Here's how the part is built. I have some questions about the finished solid (model axes, mm). A direction names the side the tool comes from. Round coordinates to 2 decimals unless told otherwise and drop trailing zeros. Write each loop counter-clockwise with the first axis right and the second up, starting at its lowest first coordinate (ties: lowest second). Pieces come first, ordered by that corner, then holes. Notation, with made-up numbers: M 27.5,53.25 L 31.5,53.25 A34 ccw 31.5,83.25 Z; hole C 40,-15.75 d6. An arc over 180 degrees is marked long. Write item = value, one per line. Start each with the question number.
(1) I want a section at C-C (y = -13). List the corners of the cut face in (x, z) for me.
(2) I want a section at D-D (z = 4). List the corners of the cut face in (x, y) for me, and give its area (3 significant figures).
(3) I need wall thicknesses on line 1 along X through (y, z) = (-9.5, 8.5); line 2 along X through (y, z) = (-25.5, 5.5); line 3 along Y through (x, z) = (-3, 8.25). Which ranges of each line are inside material? Lowest first, please.
(4) I want a section at B-B (x = 6.5). List the corners of the cut face in (y, z) for me, and give its area (3 significant figures).
(5) I want a section at A-A (z = 8.5). List the corners of the cut face in (x, y) for me, and give its area (3 significant figures).
(6) Will these pins go through, and if not, where does the flat tip stop? pin 1 Ø5 at (x, y) = (36.5, -15.5) entering from +Z; pin 2 Ø1.5 at (x, z) = (26, 5.5) entering from -Y; pin 3 Ø4 at (x, z) = (-6, 1.5) entering from +Y.
(7) If we mould it in two halves opening along X, with no side actions, what happens to faces 4 (the flat face through (-10.06, -39.96, 4.93)), 5 (the flat face through (27.17, -20.175, 7.465)), 6 (the flat face through (19, -15, 0))? For each: released by +X, released by -X, zero draft, split by the parting line, or undercut.
(8) On a 3-axis mill with a long thin cutter (end or side, diameter ignored), from which of +Z, -Z, +X, -X, +Y, -Y can I reach the whole of each face in a straight line? I mean faces 1 (the cylindrical face through (38.06, 5.15, 7.46)), 2 (the flat face through (-4.071, -45.963, 4.93)), 3 (the flat face through (16, -18, 10)). Say none if no direction works.
```python
from build123d import *

# Parameters (mm, degrees)
F1_DEPTH = 5
F2_DEPTH = 10
F3_R     = 1.9
F4_DEPTH = 25


with BuildPart() as f1:
    # F0 (on Top) → F1 (new body)
    with BuildSketch(Plane.XY):
        with BuildLine():
            Line((-12.9404729232, -48.7634912133), (5.0499415956, -43.0823117495))
            ThreePointArc((5.0499415956, -43.0823117495), (42.5104539856, 8.7293731877), (-7.2592892684, -31.4043201506))
            Line((-7.2592892684, -31.4043201506), (-12.9404729232, -48.7634912133))
        make_face()
        with BuildLine():
            ThreePointArc((0, -32.0355631411), (38.897729879, 4.3948998346), (5.0499415956, -36.7698818445))
            Line((5.0499415956, -36.7698818445), (-4.1030771099, -40.2417182922))
            Line((-4.1030771099, -40.2417182922), (0, -32.0355631411))
        make_face(mode=Mode.SUBTRACT)
        with BuildLine():
            Line((-4.1030771099, -40.2417182922), (5.0499415956, -36.7698818445))
            ThreePointArc((5.0499415956, -36.7698818445), (38.897729879, 4.3948998346), (0, -32.0355631411))
            Line((0, -32.0355631411), (-4.1030771099, -40.2417182922))
        make_face()
        with BuildLine():
            ThreePointArc((31.2465075403, -29.5105911791), (14.5582264722, -23.4633274209), (4.7343205661, -8.6795864627))
            ThreePointArc((4.7343205661, -8.6795864627), (5.8933290907, -2.69414639), (11.3623663783, 0))
            Line((11.3623663783, 0), (16.096688807, -8.3639649674))
            Line((16.096688807, -8.3639649674), (12.624851428, -12.1514201164))
            ThreePointArc((12.624851428, -12.1514201164), (17.6705032305, -18.6780973296), (25.2497028559, -21.9356808811))
            Line((25.2497028559, -21.9356808811), (29.0371589363, -18.4638462961))
            Line((29.0371589363, -18.4638462961), (36.2964533269, -22.8825435042))
            ThreePointArc((36.2964533269, -22.8825435042), (35.3488593131, -27.39838094), (31.2465075403, -29.5105911791))
        make_face(mode=Mode.SUBTRACT)
        with BuildLine():
            ThreePointArc((11.3623663783, 0), (5.8933290907, -2.69414639), (4.7343205661, -8.6795864627))
            ThreePointArc((4.7343205661, -8.6795864627), (14.5582264722, -23.4633274209), (31.2465075403, -29.5105911791))
            ThreePointArc((31.2465075403, -29.5105911791), (35.3488593131, -27.39838094), (36.2964533269, -22.8825435042))
            Line((36.2964533269, -22.8825435042), (29.0371589363, -18.4638462961))
            Line((29.0371589363, -18.4638462961), (25.2497028559, -21.9356808811))
            ThreePointArc((25.2497028559, -21.9356808811), (17.6705032305, -18.6780973296), (12.624851428, -12.1514201164))
            Line((12.624851428, -12.1514201164), (16.096688807, -8.3639649674))
            Line((16.096688807, -8.3639649674), (11.3623663783, 0))
        make_face()
    extrude(amount=F1_DEPTH)

    # F0 (on Top) → F2 (join)
    with BuildSketch(Plane.XY):
        with BuildLine():
            Line((-12.9404729232, -48.7634912133), (5.0499415956, -43.0823117495))
            ThreePointArc((5.0499415956, -43.0823117495), (42.5104539856, 8.7293731877), (-7.2592892684, -31.4043201506))
            Line((-7.2592892684, -31.4043201506), (-12.9404729232, -48.7634912133))
        make_face()
        with BuildLine():
            ThreePointArc((0, -32.0355631411), (38.897729879, 4.3948998346), (5.0499415956, -36.7698818445))
            Line((5.0499415956, -36.7698818445), (-4.1030771099, -40.2417182922))
            Line((-4.1030771099, -40.2417182922), (0, -32.0355631411))
        make_face(mode=Mode.SUBTRACT)
        with BuildLine():
            ThreePointArc((11.3623663783, 0), (5.8933290907, -2.69414639), (4.7343205661, -8.6795864627))
            ThreePointArc((4.7343205661, -8.6795864627), (14.5582264722, -23.4633274209), (31.2465075403, -29.5105911791))
            ThreePointArc((31.2465075403, -29.5105911791), (35.3488593131, -27.39838094), (36.2964533269, -22.8825435042))
            Line((36.2964533269, -22.8825435042), (29.0371589363, -18.4638462961))
            Line((29.0371589363, -18.4638462961), (25.2497028559, -21.9356808811))
            ThreePointArc((25.2497028559, -21.9356808811), (17.6705032305, -18.6780973296), (12.624851428, -12.1514201164))
            Line((12.624851428, -12.1514201164), (16.096688807, -8.3639649674))
            Line((16.096688807, -8.3639649674), (11.3623663783, 0))
        make_face()
    extrude(amount=F2_DEPTH)

    # F3 (on face) → F4 (cut)
    with BuildSketch(Plane.XY.offset(10)):
        with Locations((22.6168166846, 14.3952518702)):
            Circle(F3_R)
    extrude(amount=-F4_DEPTH, mode=Mode.SUBTRACT)


solid = f1.part
```
Returned:
q1.outline = M -11.9,0 L 52.52,0 L 52.52,10 L 47.26,10 L 47.26,5 L 13.02,5 L 13.02,10 L 6.31,10 L 6.31,5 L -5.99,5 L -5.99,10 L -11.9,10 Z
q2.outline = M -12.94,-48.76 L 5.05,-43.08 A32.25 ccw long -7.26,-31.4 Z; hole C 22.62,14.4 d3.8
q2.area = 3,380 mm²
q3.line_1 = -11.52 to -5.48, 4.97 to 15.06, 46.75 to 52.15
q3.line_2 = -10.07 to -3.95, 17.52 to 36.27, 45.22 to 50.69
q3.line_3 = -45.62 to -39.82, -38.04 to -27.52, -2.66 to 7.62
q4.outline = M -43.81,0 L 14.48,0 L 14.48,10 L 7.57,10 L 7.57,5 L -2,5 L -2,10 L -13.41,10 L -13.41,5 L -37.74,5 L -37.74,10 L -43.81,10 Z
q4.area = 413 mm²
q5.outline = M -12.94,-48.76 L 5.05,-43.08 A32.25 ccw long -7.26,-31.4 Z; M 4.73,-8.68 A28.36 ccw 31.25,-29.51 A5.37 ccw 36.3,-22.88 L 29.04,-18.46 L 25.25,-21.94 A16.45 cw 12.62,-12.15 L 16.1,-8.36 L 11.36,0 A6.85 ccw Z; hole M -4.1,-40.24 L 5.05,-36.77 A26.7 ccw long 0,-32.04 Z; hole C 22.62,14.4 d3.8
q5.area = 1,440 mm²
q6.pin_1 = 5
q6.pin_2 = -46.54
q6.pin_3 = 6.52
q7.face_4 = released by -X
q7.face_5 = undercut
q7.face_6 = zero draft
q8.face_1 = +Z
q8.face_2 = +Z, -Z, -Y
q8.face_3 = +Z, +X, -X, +Y, -Y
